Autodesk Inventor part; units mm, degrees
ref_plane "YZ Plane" through (0, 0, 0) normal (1, 0, 0) x (0, 1, 0)
ref_plane "XZ Plane" through (0, 0, 0) normal (0, 1, 0) x (-1, 0, 0)
ref_plane "XY Plane" through (0, 0, 0) normal (0, 0, 1) x (1, 0, 0)
sketch "Sketch1" plane through (0, 0, 0) normal (0, 0, 1) x (1, 0, 0)
  circle A0 centre (0, 0) radius 38.1
  dimension "d0" = 76.2
extrude "Extrusion1" add sketch "Sketch1" along normal blind 177.8
sketch "Sketch2" plane through (0, 0, 177.8) normal (0, 0, 1) x (1, 0, 0)
  circle A0 centre (0, 0) radius 38.1
  circle A1 centre (0, 0) radius 12.7
  dimension "d3" = 25.4
extrude "Extrusion2" add sketch "Sketch2" along normal blind 12.7 and the other way blind 190.5 contours A1
properties part number "Shooter_LowerMotor"
Verification items for the finished model (mm, model axes). A direction names the side the tool comes from. Coordinates: 2 decimals unless noted, no trailing zeros. Loops run counter-clockwise (first coordinate to the right, second up) from the corner with the lowest first, then second, coordinate; pieces in that order, holes last. Notation, with made-up numbers: (-37.75, 64) - (4.25, 64) arc R20 ccw to (4.25, 76) - close; hole circle Ø9 at (-8, 44.25). An arc over 180 degrees is marked (long way). Put each result on its own line as item: value.
Item 1: Scan lines: line 1 along Z through (x, y) = (16.5, -32.5); line 2 along X through (y, z) = (-1.5, 23); line 3 along Y through (x, z) = (-1, 103.5). Record each from-to range of solid material in increasing order.
Conclusion:
line 1: z = 0 to 177.8
line 2: x = -38.07 to 38.07
line 3: y = -38.09 to 38.09
Item 2: Section check A-A (x = 0). Enter the section's corners in (y, z), then the cut area to 3 significant figures.
Conclusion:
outline: (-38.1, 0) - (-12.7, 0) - (-12.7, -12.7) - (12.7, -12.7) - (12.7, 0) - (38.1, 0) - (38.1, 177.8) - (12.7, 177.8) - (12.7, 190.5) - (-12.7, 190.5) - (-12.7, 177.8) - (-38.1, 177.8) - close
area: 14,200 mm2
Item 3: Section check C-C (z = 29.5). Enter the section's corners in (x, y).
Conclusion:
outline: circle Ø76.2 at (0, 0)
Item 4: Set-up check for faces 1 (the face through (-2.75, -12.4, -6.26)), 2 (the face through (16, 1, 177.8)), 3 (the face through (0, 0, 190.5)): record each of +Z, -Z, +X, -X, +Y, -Y from which the full face is reachable in a straight line by a thin tool's end or side.
Conclusion:
face 1: -Z
face 2: +Z
face 3: +Z, +X, -X, +Y, -Y
Item 5: Section check D-D (y = -29). Enter the section's corners in (x, z), then the cut area to 3 significant figures.
Conclusion:
outline: (-24.71, 0) - (24.71, 0) - (24.71, 177.8) - (-24.71, 177.8) - close
area: 8,790 mm2
Item 6: Gauge pin test, flat ends, axial feed: pin 1 Ø6 at (x, y) = (8, 21.5) entering from -Z; pin 2 Ø5 at (x, y) = (-14, 2) entering from +Z; pin 3 Ø1 at (y, z) = (-6, 36) entering from -X; pin 4 Ø1.5 at (y, z) = (1.5, 113.5) entering from +X. Record the tip position at first contact, or that the pin passes through.
Conclusion:
pin 1: stops at z = 0
pin 2: stops at z = 190.5
pin 3: stops at x = -37.7
pin 4: stops at x = 38.09
